from build123d import *

# Parameters (mm, degrees)
CROQUIS1_W              = 14
CROQUIS1_H              = 25
SALIENTE_EXTRUIR1_DEPTH = 200
REDONDEO1_R             = 10
REDONDEO2_R             = 10
CROQUIS2_R              = 8.6
CORTAR_EXTRUIR1_DEPTH   = 28
CROQUIS14_R             = 9.913044
SALIENTE_EXTRUIR2_DEPTH = 14
CROQUIS12_R             = 2
CORTAR_EXTRUIR7_DEPTH   = 203.042074826
CROQUIS15_W             = 3
CROQUIS15_H             = 5.6
CORTAR_EXTRUIR9_DEPTH   = 8
CROQUIS16_W             = 17
CROQUIS16_H             = 145
CORTAR_EXTRUIR10_DEPTH  = 4
CROQUIS17_W             = 17
CROQUIS17_H             = 145
CORTAR_EXTRUIR11_DEPTH  = 4
REDONDEO5_R             = 2
REDONDEO6_R             = 2
CROQUIS18_W             = 1
CROQUIS18_H             = 1
CORTAR_EXTRUIR12_DEPTH  = 203.042074845
CROQUIS19_W             = 6
CROQUIS19_H             = 25
SALIENTE_EXTRUIR3_DEPTH = 50
CROQUIS20_R             = 8.6
CORTAR_EXTRUIR13_DEPTH  = 6
REDONDEO7_R             = 10
REDONDEO8_R             = 10
REDONDEO9_R             = 10
REDONDEO10_R            = 10
REDONDEO11_R            = 10
REDONDEO12_R            = 10


with BuildPart() as part:
    # Croquis1 → Saliente-Extruir1 (new body)
    with BuildSketch(Plane(origin=(0, 0, 0), x_dir=(1, 0, 0), z_dir=(0, 1, 0))):
        with Locations((7, 12.5)):
            Rectangle(CROQUIS1_W, CROQUIS1_H)
    extrude(amount=SALIENTE_EXTRUIR1_DEPTH)

    # Redondeo1
    redondeo1_edges = [part.edges().sort_by_distance(p)[0] for p in [
        (7, 0, -25),
    ]]
    fillet(redondeo1_edges, radius=REDONDEO1_R)

    # Redondeo2
    redondeo2_edges = [part.edges().sort_by_distance(p)[0] for p in [
        (7, 0, 0),
    ]]
    fillet(redondeo2_edges, radius=REDONDEO2_R)

    # Croquis2 → Cortar-Extruir1 (cut)
    with BuildSketch(Plane(origin=(14, 0, 0), x_dir=(0, 0, -1), z_dir=(1, 0, 0))):
        with Locations((12.5, 12.5)):
            Circle(CROQUIS2_R)
        with BuildLine():
            Line((10.5, 185.263932023), (10.5, 189.736067977))
            ThreePointArc((10.5, 189.736067977), (15.5, 187.5), (10.5, 185.263932023))
        make_face()
    extrude(amount=-CORTAR_EXTRUIR1_DEPTH, mode=Mode.SUBTRACT)

    # Croquis14 → Saliente-Extruir2 (add)
    with BuildSketch(Plane(origin=(14, 0, 0), x_dir=(0, 0, -1), z_dir=(1, 0, 0))):
        with Locations((12.5, 187.5)):
            Circle(CROQUIS14_R)
        with BuildLine():
            Line((10.5, 185.263932023), (10.5, 189.736067977))
            ThreePointArc((10.5, 189.736067977), (15.5, 187.5), (10.5, 185.263932023))
        make_face(mode=Mode.SUBTRACT)
    extrude(amount=-SALIENTE_EXTRUIR2_DEPTH)

    # Croquis12 → Cortar-Extruir7 (cut, through all)
    with BuildSketch(Plane(origin=(0, 0, -25), x_dir=(-1, 0, 0), z_dir=(0, 0, -1))):
        with Locations((-4, 187.5)):
            Circle(CROQUIS12_R)
    extrude(amount=-CORTAR_EXTRUIR7_DEPTH, mode=Mode.SUBTRACT)

    # Croquis15 → Cortar-Extruir9 (cut)
    with BuildSketch(Plane.ZY):
        with Locations((-6.582205818, 187.5)):
            Rectangle(CROQUIS15_W, CROQUIS15_H)
    extrude(amount=-CORTAR_EXTRUIR9_DEPTH, mode=Mode.SUBTRACT)

    # Croquis16 → Cortar-Extruir10 (cut)
    with BuildSketch(Plane.ZY):
        with Locations((-12.5, 97.5)):
            Rectangle(CROQUIS16_W, CROQUIS16_H)
    extrude(amount=-CORTAR_EXTRUIR10_DEPTH, mode=Mode.SUBTRACT)

    # Croquis17 → Cortar-Extruir11 (cut)
    with BuildSketch(Plane(origin=(14, 0, 0), x_dir=(0, 0, -1), z_dir=(1, 0, 0))):
        with Locations((12.5, 97.5)):
            Rectangle(CROQUIS17_W, CROQUIS17_H)
    extrude(amount=-CORTAR_EXTRUIR11_DEPTH, mode=Mode.SUBTRACT)

    # Redondeo5
    redondeo5_edges = [part.edges().sort_by_distance(p)[0] for p in [
        (4, 97.5, -21),
        (4, 170, -12.5),
        (4, 97.5, -4),
        (4, 25, -12.5),
    ]]
    fillet(redondeo5_edges, radius=REDONDEO5_R)

    # Redondeo6
    redondeo6_edges = [part.edges().sort_by_distance(p)[0] for p in [
        (10, 97.5, -21),
        (10, 25, -12.5),
        (10, 97.5, -4),
        (10, 170, -12.5),
    ]]
    fillet(redondeo6_edges, radius=REDONDEO6_R)

    # Croquis18 → Cortar-Extruir12 (cut, through all)
    with BuildSketch(Plane(origin=(14, 0, 0), x_dir=(0, 0, -1), z_dir=(1, 0, 0))):
        with Locations((12.5, 199.5)):
            Rectangle(CROQUIS18_W, CROQUIS18_H)
    extrude(amount=-CORTAR_EXTRUIR12_DEPTH, mode=Mode.SUBTRACT)

    # Croquis19 → Saliente-Extruir3 (add)
    with BuildSketch(Plane(origin=(0, 200, 0), x_dir=(1, 0, 0), z_dir=(0, 1, 0))):
        with Locations((7, 12.5)):
            Rectangle(CROQUIS19_W, CROQUIS19_H)
    extrude(amount=SALIENTE_EXTRUIR3_DEPTH)

    # Croquis20 → Cortar-Extruir13 (cut)
    with BuildSketch(Plane(origin=(10, 0, 0), x_dir=(0, 0, -1), z_dir=(1, 0, 0))):
        with Locations((12.5, 237.5)):
            Circle(CROQUIS20_R)
    extrude(amount=-CORTAR_EXTRUIR13_DEPTH, mode=Mode.SUBTRACT)

    # Redondeo7
    redondeo7_edges = [part.edges().sort_by_distance(p)[0] for p in [
        (7, 250, 0),
    ]]
    fillet(redondeo7_edges, radius=REDONDEO7_R)

    # Redondeo8
    redondeo8_edges = [part.edges().sort_by_distance(p)[0] for p in [
        (7, 250, -25),
    ]]
    fillet(redondeo8_edges, radius=REDONDEO8_R)

    # Redondeo9
    redondeo9_edges = [part.edges().sort_by_distance(p)[0] for p in [
        (2, 200, 0),
    ]]
    fillet(redondeo9_edges, radius=REDONDEO9_R)

    # Redondeo10
    redondeo10_edges = [part.edges().sort_by_distance(p)[0] for p in [
        (12, 200, 0),
    ]]
    fillet(redondeo10_edges, radius=REDONDEO10_R)

    # Redondeo11
    redondeo11_edges = [part.edges().sort_by_distance(p)[0] for p in [
        (12, 200, -25),
    ]]
    fillet(redondeo11_edges, radius=REDONDEO11_R)

    # Redondeo12
    redondeo12_edges = [part.edges().sort_by_distance(p)[0] for p in [
        (2, 200, -25),
    ]]
    fillet(redondeo12_edges, radius=REDONDEO12_R)


solid = part.part
Check sheet for the modelled part. Datum: model origin and axes. Units: mm. A direction names the side the tool comes from. Give positions to 0.01 mm unless a question says otherwise; leave off trailing zeros. Loops run counter-clockwise (first coordinate to the right, second up) from the corner with the lowest first, then second, coordinate; pieces in that order, holes last. Notation, with made-up numbers: M 50,-26.75 L 101,-26.75 A14 ccw 101,-10.75 Z; hole C 36,-9.5 d3. An arc over 180 degrees is marked long. Answer as a JSON object with one key per item and string values. Group by question number.
Q1. Access from +Z, -Z, +X, -X, +Y, -Y to the whole of each face (thin tool, end or side, straight path). Record for faces 1 (the cylindrical face through (12.03, 197.15, -3.01)), 2 (the flat face through (4, 98, -13)), 3 (the flat face through (10, 98, -12)).
Q2. Go/stop test with flat-tipped pins: P1, Ø1, axis at x = 3, z = -11, coming from the +Y side; P2, Ø4, axis at x = 5.5, z = -22.5, coming from the +Y side; P3, Ø4, axis at x = 6.5, z = -22, coming from the -Y side. Record where each tip stops, or that it passes through.
Q3. Material ranges on line 1 along Y through (x, z) = (5, -12.5); line 2 along Y through (x, z) = (12.25, -11.5); line 3 along X through (y, z) = (187.5, -2.8), recorded low to high. Write a range as [from, to].
Q4. Cross-section at C-C on y = 237.5. Record the cut outline in (x, z), then the cut area to 3 significant figures.
Q5. Cross-section at B-B on y = 142. Record the cut outline in (x, z).
Q6. Cross-section at A-A on y = 12.5. Record the cut outline in (x, z), then the cut area to 3 significant figures.
Q7. Release check for a two-part mould opening along Z. For faces 4 (the flat face through (7, 250, -13)), 5 (the cylindrical face through (7.1, 12.88, -3.91)), 6 (the cylindrical face through (12.03, 197.15, -21.99)) record: released by +Z, released by -Z, zero draft, split by the parting line, or undercut.
Evaluation:
{
 "1": {"face 1": "+Z, +X, +Y", "face 2": "-X", "face 3": "+X"},
 "2": {"P1": "stops at y = 200", "P2": "stops at y = 248.35", "P3": "stops at y = 1.34"},
 "3": {"line 1": "y = [0, 3.9], [21.1, 184.5], [190.5, 199], [200, 228.9], [246.1, 250]", "line 2": "y = [0, 3.96], [21.04, 25], [170, 184.67], [190.33, 200]", "line 3": "x = [0, 2], [6, 14]"},
 "4": {"outline": "M 4,-25 L 10,-25 L 10,-21.1 L 4,-21.1 Z; M 4,-3.9 L 10,-3.9 L 10,0 L 4,0 Z", "area": "46.8 mm2"},
 "5": {"outline": "M 0,-25 L 14,-25 L 14,-21 L 12,-21 A2 cw 10,-19 L 10,-6 A2 cw 12,-4 L 14,-4 L 14,0 L 0,0 L 0,-4 L 2,-4 A2 cw 4,-6 L 4,-19 A2 cw 2,-21 L 0,-21 Z"},
 "6": {"outline": "M 0,-25 L 14,-25 L 14,-21.1 L 0,-21.1 Z; M 0,-3.9 L 14,-3.9 L 14,0 L 0,0 Z", "area": "109 mm2"},
 "7": {"face 4": "zero draft", "face 5": "undercut", "face 6": "released by -Z"}
}
